Check sheet for the modelled part. Datum: model origin and axes. Units: mm. A direction names the side the tool comes from. Coordinates: 2 decimals unless noted, no trailing zeros. Loops run counter-clockwise (first coordinate to the right, second up) from the corner with the lowest first, then second, coordinate; pieces in that order, holes last. Notation, with made-up numbers: (39, -3) - (83, -3) arc R30 ccw to (83, 33) - close; hole circle Ø9 at (82, 53). An arc over 180 degrees is marked (long way). Write each question's results on one line, items separated by ' | '. Start each with the question number.
1. Thickness scan on line 1 (Z direction, x = -52.5, y = -44.5); line 2 (Y direction, x = 0, z = 55); line 3 (Y direction, x = -110, z = -5). Record the ranges inside material, lowest first. Write a range as [from, to].
2. Gauge pin test, flat ends, axial feed: P1, Ø4, axis at y = -18, z = 57, coming from the -X side; P2, Ø18, axis at x = 0, y = 0, coming from the +Z side; P3, Ø6, axis at x = -11.5, z = 58, coming from the -Y side; P4, Ø3, axis at x = 3, y = -25.5, coming from the +Z side. Record the tip position at first contact, or that the pin passes through.
3. Cross-section at C-C (x = 0). Record the cut outline in (y, z), and give its area (3 significant figures).
4. Cross-section at B-B (y = -44). Record the cut outline in (x, z).
5. Draft check along Z on faces 1 (the face through (30, -27, 39)), 2 (the face through (-65, -16, 32)), 3 (the face through (-51, -42, 38)), 4 (the face through (-65, -16, 44)). Enter one of: released by +Z, released by -Z, zero draft, split by the parting line, or undercut.
6. Cross-section at D-D (z = 2). Record the cut outline in (x, y).
7. Tool access check on faces 5 (the face through (-51, -42, 82)), 6 (the face through (-21, -14, 0)), 7 (the face through (-51, -48, 12)), 8 (the face through (-30, -15, 16)). Record the directions out of +Z, -Z, +X, -X, +Y, -Y that give a thin tool (end or side, any length) a straight path to the whole face; none if there is none.
8. Cross-section at A-A (z = 25.5). Record the cut outline in (x, y).
```python
from build123d import *

# Parameters (mm, degrees)
SKETCH1_R           = 15
BOSS_EXTRUDE1_DEPTH = 76
SKETCH2_W           = 160
SKETCH2_H           = 24
BOSS_EXTRUDE2_DEPTH = 12
RIB1_START          = -6
RIB1_DEPTH          = 12


# Read off the part's stored shape, not the designer's step: Rib1
with BuildPart() as part:
    # Sketch1 → Boss-Extrude1 (new body)
    with BuildSketch(Plane.XY):
        with BuildLine():
            Line((-30, 0), (-30, -30))
            Line((-30, -30), (-130, -30))
            Line((-130, -30), (-130, -42))
            Line((-130, -42), (30, -42))
            Line((30, -42), (30, 0))
            ThreePointArc((30, 0), (0, 30), (-30, 0))
        make_face()
        Circle(SKETCH1_R, mode=Mode.SUBTRACT)
    extrude(amount=BOSS_EXTRUDE1_DEPTH)

    # Sketch2 → Boss-Extrude2 (add)
    with BuildSketch(Plane.XZ.offset(42)):
        with Locations((-50, 76)):
            Rectangle(SKETCH2_W, SKETCH2_H)
    boss_extrude2 = extrude(amount=BOSS_EXTRUDE2_DEPTH)

    # Mirror1: Boss-Extrude2 across plane
    add(boss_extrude2.mirror(Plane.XY.offset(38)))

    # Rib1 outline → Rib1 (add)
    with BuildSketch(Plane.XY.offset(38).offset(RIB1_START)):
        with BuildLine():
            Line((-22.829268293, 19.463414634), (-130, -30))
            Line((-130, -30), (-30, -30))
            Line((-30, -30), (-30, 0))
            ThreePointArc((-30, 0), (-28.150293505, 10.371160765), (-22.829268293, 19.463414634))
        make_face()
    extrude(amount=RIB1_DEPTH)


solid = part.part
```
Established:
1) line 1: [-12, 12], [64, 88] | line 2: [-42, -15], [15, 30] | line 3: [-54, -42]
2) P1: x = -30 | P2: through | P3: y = -42 | P4: z = 76
3) outline: (-54, -12) - (-42, -12) - (-42, 0) - (-15, 0) - (-15, 76) - (-42, 76) - (-42, 88) - (-54, 88) - (-54, 64) - (-42, 64) - (-42, 12) - (-54, 12) - close; (15, 0) - (30, 0) - (30, 76) - (15, 76) - close | area: 3,770 mm^2
4) outline: (-130, -12) - (30, -12) - (30, 12) - (-130, 12) - close; (-130, 64) - (30, 64) - (30, 88) - (-130, 88) - close
5) face 1: zero draft | face 2: released by -Z | face 3: undercut | face 4: released by +Z
6) outline: (-130, -54) - (30, -54) - (30, 0) arc R30 ccw to (-30, 0) - (-30, -30) - (-130, -30) - close; hole circle Ø30 at (0, 0)
7) face 5: +Z, +X, -X, +Y | face 6: -Z, +X, -X, +Y | face 7: +X, -X, -Y | face 8: -Z, -X, +Y
8) outline: (-130, -42) - (30, -42) - (30, 0) arc R30 ccw to (-30, 0) - (-30, -30) - (-130, -30) - close; hole circle Ø30 at (0, 0)
